```python
from build123d import *

# Parameters (mm, degrees)
BOSS_EXTRUDE2_START        = 2
SKETCH1_W                  = 12.4
SKETCH1_H                  = 22.6
BOSS_EXTRUDE2_DEPTH        = 27
SKETCH2_W                  = 7.2
SKETCH2_H                  = 2.1
CUT_EXTRUDE1_DEPTH         = 7.5
SKETCH3_W                  = 12.4
SKETCH3_H                  = 11
CUT_EXTRUDE2_DEPTH         = 124.829883308
CUT_EXTRUDE2_DEPTH_BACK    = 124.829883308
SKETCH2_3_W                = 7.2
SKETCH2_3_H                = 6
CUT_EXTRUDE3_DEPTH         = 10
SKETCH7_R                  = 1.05
SKETCH7_R_2                = 1.5
CUT_EXTRUDE9_DEPTH         = 124.829883308
SKETCH1_8_R                = 1.5
CUT_EXTRUDE12_DEPTH        = 12
F_2_2_2_2_DIAMETER_HOLE1_D = 2.2


with BuildPart() as part:
    # Sketch1 → Boss-Extrude2 (new body)
    with BuildSketch(Plane(origin=(0, 0, 0), x_dir=(1, 0, 0), z_dir=(0, 1, 0)).offset(BOSS_EXTRUDE2_START)):
        Polygon((84, 98), (84, 77), (116, 77), (116, 98), (108.8, 98), (108.8, 109.2), (91.2, 109.2), (91.2, 98), align=None)
        with Locations((100, 93.1)):
            Rectangle(SKETCH1_W, SKETCH1_H, mode=Mode.SUBTRACT)
    extrude(amount=BOSS_EXTRUDE2_DEPTH)

    # Sketch2 → Cut-Extrude1 (cut)
    with BuildSketch(Plane(origin=(0, 29, 0), x_dir=(1, 0, 0), z_dir=(0, 1, 0))):
        with Locations((112.4, 78.05)):
            Rectangle(SKETCH2_W, SKETCH2_H)
        Polygon((84, 79.1), (84, 78.995319666), (84, 77), (91.2, 77), (91.2, 79.1), align=None)
    extrude(amount=-CUT_EXTRUDE1_DEPTH, mode=Mode.SUBTRACT)

    # Sketch3 → Cut-Extrude2 (cut, two sides)
    with BuildSketch(Plane.XY.offset(-77)) as cut_extrude2_sk:
        with Locations((100, 7.5)):
            Rectangle(SKETCH3_W, SKETCH3_H)
    extrude(amount=CUT_EXTRUDE2_DEPTH, mode=Mode.SUBTRACT)
    extrude(cut_extrude2_sk.sketch, amount=-CUT_EXTRUDE2_DEPTH_BACK, mode=Mode.SUBTRACT)

    # Sketch2<3> → Cut-Extrude3 (cut)
    with BuildSketch(Plane(origin=(0, 29, 0), x_dir=(1, 0, 0), z_dir=(0, 1, 0))):
        Polygon((108.8, 84.5), (116, 84.5), (116, 85.211636412), (116, 90.5), (108.8, 90.5), align=None)
        with Locations((87.6, 87.5)):
            Rectangle(SKETCH2_3_W, SKETCH2_3_H)
    extrude(amount=-CUT_EXTRUDE3_DEPTH, mode=Mode.SUBTRACT)

    # Sketch7 → Cut-Extrude9 (cut, through all)
    with BuildSketch(Plane.XY.offset(-77)):
        with Locations((87.5, 25.25)):
            Circle(SKETCH7_R)
        with Locations((112.5, 25.25)):
            Circle(SKETCH7_R)
        with Locations((87.5, 5.5)):
            Circle(SKETCH7_R_2)
        with Locations((112.5, 5.5)):
            Circle(SKETCH7_R_2)
    extrude(amount=-CUT_EXTRUDE9_DEPTH, mode=Mode.SUBTRACT)

    # Sketch1<8> → Cut-Extrude12 (cut)
    with BuildSketch(Plane(origin=(0, 0, 0), x_dir=(1, 0, 0), z_dir=(0, 1, 0))):
        with Locations(Location((109, 82, 0), (0, 0, 270))):
            Circle(SKETCH1_8_R)
        with Locations(Location((109, 93, 0), (0, 0, 270))):
            Circle(SKETCH1_8_R)
        with Locations(Location((91, 82, 0), (0, 0, 270))):
            Circle(SKETCH1_8_R)
        with Locations(Location((91, 93, 0), (0, 0, 270))):
            Circle(SKETCH1_8_R)
    extrude(amount=CUT_EXTRUDE12_DEPTH, mode=Mode.SUBTRACT)

    # Ø2.2 (2.2) Diameter Hole1 (through all)
    with Locations(Plane(origin=(0, 29, 0), x_dir=(1, 0, 0), z_dir=(0, 1, 0))):
        with Locations((100, 79.2), (100, 107)):
            Hole(F_2_2_2_2_DIAMETER_HOLE1_D / 2)


solid = part.part
```
CAD build for the part. Positions are in the model's coordinates, mm. A direction names the side the tool comes from. Give positions to 0.01 mm unless a question says otherwise; leave off trailing zeros. Order: outer loops, then holes, each group sorted by start corner. A loop starts at its lowest first (then second) coordinate and runs counter-clockwise, first axis right, second up.
(1) Saw through at D-D, the plane z = -107. Give the cut face in (x, y), then the cut area to 3 significant figures.
(2) Tool access for faces 1 (the flat face through (109, 12, -82)), 2 (the flat face through (112, 24, -84.5)), 3 (the flat face through (100, 21, -81.8)), 4 (the flat face through (88, 19, -88)), 5 (the flat face through (88.5, 26.1, -79.1)): list every direction of +Z, -Z, +X, -X, +Y, -Y with a clear straight run to the whole face (end or side of a thin tool).
(3) Drill centre lines: L1, parallel to X at y = 19.75, z = -79.2; L2, parallel to X at y = 12.75, z = -79; L3, parallel to Z at x = 99.5, y = 19.25. Where is each one in solid material? Low to high.
(4) Flat gauge pins, fed straight in: pin 1 (0.9 mm diameter, centred on x = 91.5, z = -92.5, fed in from -Y); pin 2 (1 mm diameter, centred on y = 27, z = -77.5, fed in from +X); pin 3 (8 mm diameter, centred on x = 87, y = 27, fed in from +Z). Where does each tip first touch, or does it go through?
(5) Saw through at B-B, the plane z = -96. Give the cut face in (x, y), then the cut area to 3 significant figures.
(6) Saw through at C-C, the plane x = 97. Give the cut face in (y, z), then the cut area to 3 significant figures.
(7) Mould opens along X. For faces 6 (the flat face through (100, 21, -104.4)), 7 (the flat face through (91.2, 15, -104)), 8 (the flat face through (108.8, 24, -88)) say: released by +X, released by -X, zero draft, split by the parting line, or undercut.
(8) Saw through at A-A, the plane y = 5.5. Give the cut face in (x, z).
Results found:
1. outline: (91.2, 2) - (93.8, 2) - (93.8, 13) - (98.9, 13) - (98.9, 29) - (91.2, 29) - close; (101.1, 13) - (106.2, 13) - (106.2, 2) - (108.8, 2) - (108.8, 29) - (101.1, 29) - close
1. area: 304 mm2
2. face 1: -Y
2. face 2: +X, +Y
2. face 3: +Y, -Y
2. face 4: -X, +Y
2. face 5: +Z, -X, +Y
3. L1: x = 84 to 98.9, 101.1 to 116
3. L2: x = 84 to 93.8, 106.2 to 116
3. L3: z = -109.2 to -107.98, -106.02 to -104.4, -81.8 to -80.18, -78.22 to -77
4. pin 1: stops at y = 12
4. pin 2: stops at x = 108.8
4. pin 3: stops at z = -79.1
5. outline: (84, 2) - (93.8, 2) - (93.8, 29) - (84, 29) - close; (106.2, 2) - (116, 2) - (116, 29) - (106.2, 29) - close; hole circle Ø3 at (87.5, 5.5); hole circle Ø2.1 at (87.5, 25.25); hole circle Ø3 at (112.5, 5.5); hole circle Ø2.1 at (112.5, 25.25)
5. area: 508 mm2
6. outline: (13, -109.2) - (29, -109.2) - (29, -104.4) - (13, -104.4) - close; (13, -81.8) - (29, -81.8) - (29, -77) - (13, -77) - close
6. area: 154 mm2
7. face 6: undercut
7. face 7: released by -X
7. face 8: released by +X
8. outline: (84, -98) - (86, -98) - (86, -77) - (84, -77) - close; (89, -98) - (91.2, -98) - (91.2, -109.2) - (93.8, -109.2) - (93.8, -77) - (89, -77) - close; (106.2, -109.2) - (108.8, -109.2) - (108.8, -98) - (111, -98) - (111, -77) - (106.2, -77) - close; (114, -98) - (116, -98) - (116, -77) - (114, -77) - close; hole circle Ø3 at (91, -93); hole circle Ø3 at (91, -82); hole circle Ø3 at (109, -93); hole circle Ø3 at (109, -82)
